Can you work these out from the model? Positions are in its coordinate system, mm. A direction names the side the tool comes from. Coordinates: 2 decimals unless noted, no trailing zeros. Write each loop counter-clockwise with the first axis right and the second up, starting at its lowest first coordinate (ties: lowest second). Pieces come first, ordered by that corner, then holes. Notation, with made-up numbers: (-10.75, -0.5) -> (36.25, -0.5) arc R33 ccw to (36.25, 34.5) -> close; hole circle Ø8 at (63.25, -14.75). An arc over 180 degrees is marked (long way). Use one line per item in the form item = value.
```python
from build123d import *

# Parameters (mm, degrees)
SKETCH_1_R               = 8
EXTRUDE_1_DEPTH          = 630
SKETCH_2_R               = 4
CUT_EXTRUDE_1_DEPTH      = 9
CUT_EXTRUDE_1_DEPTH_BACK = 9
SKETCH_3_OUTSIDE_W       = 144.082
SKETCH_3_OUTSIDE_H       = 144.082
SKETCH_3_OUTSIDE_W_2     = 20
SKETCH_3_OUTSIDE_H_2     = 10
CUT_EXTRUDE_2_DEPTH      = 20
CUT_EXTRUDE_START        = 5
CUT_EXTRUDE_3_DEPTH      = 4


with BuildPart() as part:
    # 草图1 → 凸台-拉伸1 (new body)
    with BuildSketch(Plane(origin=(0, 0, 0), x_dir=(0, 0, -1), z_dir=(1, 0, 0))):
        Circle(SKETCH_1_R)
    extrude(amount=EXTRUDE_1_DEPTH)

    # 草图2 → 切除-拉伸1 (cut, two sides)
    with BuildSketch(Plane(origin=(0, 0, 0), x_dir=(1, 0, 0), z_dir=(0, 1, 0))) as cut_extrude_1_sk:
        with Locations((10, 0)):
            Circle(SKETCH_2_R)
    extrude(amount=CUT_EXTRUDE_1_DEPTH, mode=Mode.SUBTRACT)
    extrude(cut_extrude_1_sk.sketch, amount=-CUT_EXTRUDE_1_DEPTH_BACK, mode=Mode.SUBTRACT)

    # 草图3 outside → 切除-拉伸2 (cut)
    with BuildSketch(Plane.ZY):
        Rectangle(SKETCH_3_OUTSIDE_W, SKETCH_3_OUTSIDE_H)
        Rectangle(SKETCH_3_OUTSIDE_W_2, SKETCH_3_OUTSIDE_H_2, mode=Mode.SUBTRACT)
    extrude(amount=-CUT_EXTRUDE_2_DEPTH, mode=Mode.SUBTRACT)

    # 草图4 → 切除-拉伸3 (cut, through all)
    with BuildSketch(Plane(origin=(0, 0, 0), x_dir=(1, 0, 0), z_dir=(0, 1, 0)).offset(CUT_EXTRUDE_START)):
        with BuildLine():
            Line((475, 2.5), (575, 2.5))
            ThreePointArc((575, 2.5), (577.5, 0), (575, -2.5))
            Line((575, -2.5), (475, -2.5))
            ThreePointArc((475, -2.5), (472.5, 0), (475, 2.5))
        make_face()
    extrude(amount=CUT_EXTRUDE_3_DEPTH, mode=Mode.SUBTRACT)


solid = part.part
```
Q1. Suppose I cut it at A-A (z = 0). Write out the boundary of the cut face in (x, y), then the cut area to 4 significant figures.
Return value:
outline = (0, -5) -> (6, -5) -> (6, 5) -> (0, 5) -> close; (14, -5) -> (20, -5) -> (20, -8) -> (630, -8) -> (630, 8) -> (577.5, 8) -> (577.5, 5) -> (472.5, 5) -> (472.5, 8) -> (20, 8) -> (20, 5) -> (14, 5) -> close
area = 9,565 mm2
Q2. Suppose I cut it at B-B (y = 2.5). Write out the boundary of the cut face in (x, z).
Return value:
outline = (0, -7.6) -> (630, -7.6) -> (630, 7.6) -> (0, 7.6) -> close; hole circle Ø8 at (10, 0)
Q3. Will these pins go through, and if not, where does the flat tip stop? pin 1 (7 mm diameter, centred on x = 10, z = 0, fed in from -Y) (1 decimal); pin 2 (4 mm diameter, centred on x = 546, z = 1, fed in from +Y); pin 3 (3.5 mm diameter, centred on y = 7, z = -2.5, fed in from -X); pin 4 (0.8 mm diameter, centred on x = 511, y = 6, fed in from +Z).
Return value:
pin_1 = through
pin_2 = 7.6
pin_3 = 20
pin_4 = 5.71
Q4. Suppose I cut it at D-D (x = 140). Write out the boundary of the cut face in (y, z).
Return value:
outline = circle Ø16 at (0, 0)
Q5. Suppose I cut it at C-C (x = 540.5). Write out the boundary of the cut face in (y, z), then the cut area to 3 significant figures.
Return value:
outline = (5, -2.5) -> (5, 2.5) -> (7.6, 2.5) arc R8 ccw (long way) to (7.6, -2.5) -> close
area = 187 mm2
Q6. If I drill on line 1 (X direction, y = -2.6, z = 0); line 2 (Z direction, x = 130, y = 0.5), over which ranges is the centre line in solid material (lowest first)? Write a range as from..to.
Return value:
line_1 = 0..6, 14..630
line_2 = -7.98..7.98
Q7. For faces 1 (the flat face through (9.9, 5, -4.3)), 2 (the flat face through (9.9, -5, -4.3)), 3 (the cylindrical face through (310.59, -7.81, 1.73)), which set-ups out of +Z, -Z, +X, -X, +Y, -Y let a thin tool reach every point of the face, with its end or its side?
Return value:
face_1 = +Z, -Z, -X, +Y
face_2 = +Z, -Z, -X, -Y
face_3 = +X, -X
